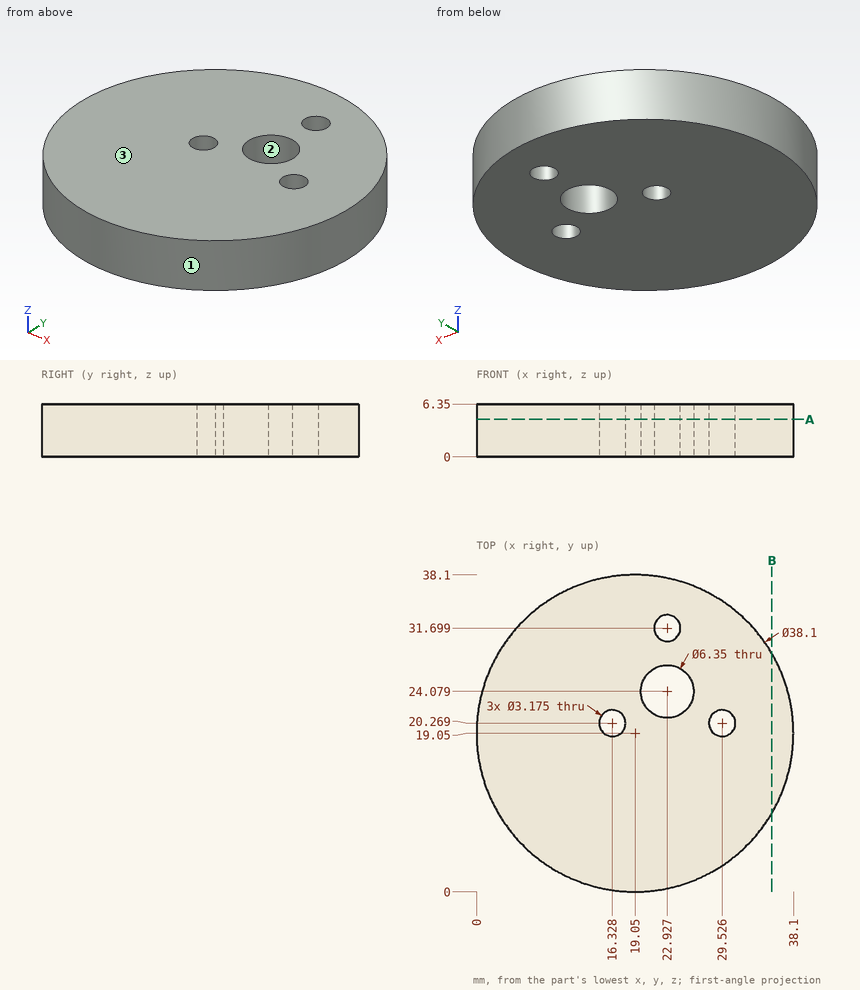
Here's the drawing with two shaded views (mm, measured from the low corner). I have some questions. Coordinates: 2 decimals unless noted, no trailing zeros. Order: outer loops, then holes, each group sorted by start corner. A loop starts at its lowest first (then second) coordinate and runs counter-clockwise, first axis right, second up. Notation, with made-up numbers: (59, 43) - (68, 43) arc R16 ccw to (68, 51) - close; hole circle Ø5 at (21, -6.5). An arc over 180 degrees is marked (long way). Use CSV: the item, a comma, the result in double quotes. Start each with the question number.
1. Please list where these lines run through material, in increasing order: line 1 (X direction, y = 21.5, z = 1) (1 decimal); line 2 (Y direction, x = 22.5, z = 2.25) (1 decimal); line 3 (Y direction, x = 21.5, z = 5.75) (1 decimal). Write a range as from..to.
2. I'm going to push flat-ended pins straight in: pin 1 (5 mm diameter, centred on x = 7, y = 9, fed in from -Z); pin 2 (1.5 mm diameter, centred on y = 9, z = 4.5, fed in from -X) (1 decimal). Where does each tip first touch, or does it pass through?
3. Suppose I cut it at A-A on z = 4.5. Give the number of separate pieces and of enclosed holes in the cut face, then the cut area to 3 significant figures.
4. If we mould it in two halves opening along Y, with no side actions, what happens to the marked faces 1, 2 and 3? For each: +Y half, -Y half, draft (parallel to the pull), parting line (faces both ways), or undercut.
5. Suppose I cut it at B-B on x = 35.5. List the corners of the cut face in (y, z) for me.
Output:
1,line 1,"x = 0.2..15.3, 17.3..21.1, 24.8..28.5, 30.5..37.9"
1,line 2,"y = 0.3..20.9, 27.2..30.2, 33.2..37.8"
1,line 3,"y = 0.2..21.2, 26.9..31, 32.4..37.9"
2,pin 1,"stops at z = 0"
2,pin 2,"stops at x = 2.4"
3,separate pieces,"1"
3,enclosed holes,"4"
3,area,"1,080 mm2"
4,face 1,"parting line"
4,face 2,"undercut"
4,face 3,"draft"
5,outline,"(9.44, 0) - (28.66, 0) - (28.66, 6.35) - (9.44, 6.35) - close"
